For this review, use the dimensioned drawing (mm, ordinates from the lowest corner) and the shaded views. Give positions to 0.01 mm unless a question says otherwise; leave off trailing zeros. Loops run counter-clockwise (first coordinate to the right, second up) from the corner with the lowest first, then second, coordinate; pieces in that order, holes last. Notation, with made-up numbers: M -31.75,69.5 L -7.75,69.5 A29 cw -7.75,92.5 Z; hole C -13,9.5 d8. An arc over 180 degrees is marked long. Use CSV: the item, a comma, the result in double quotes.
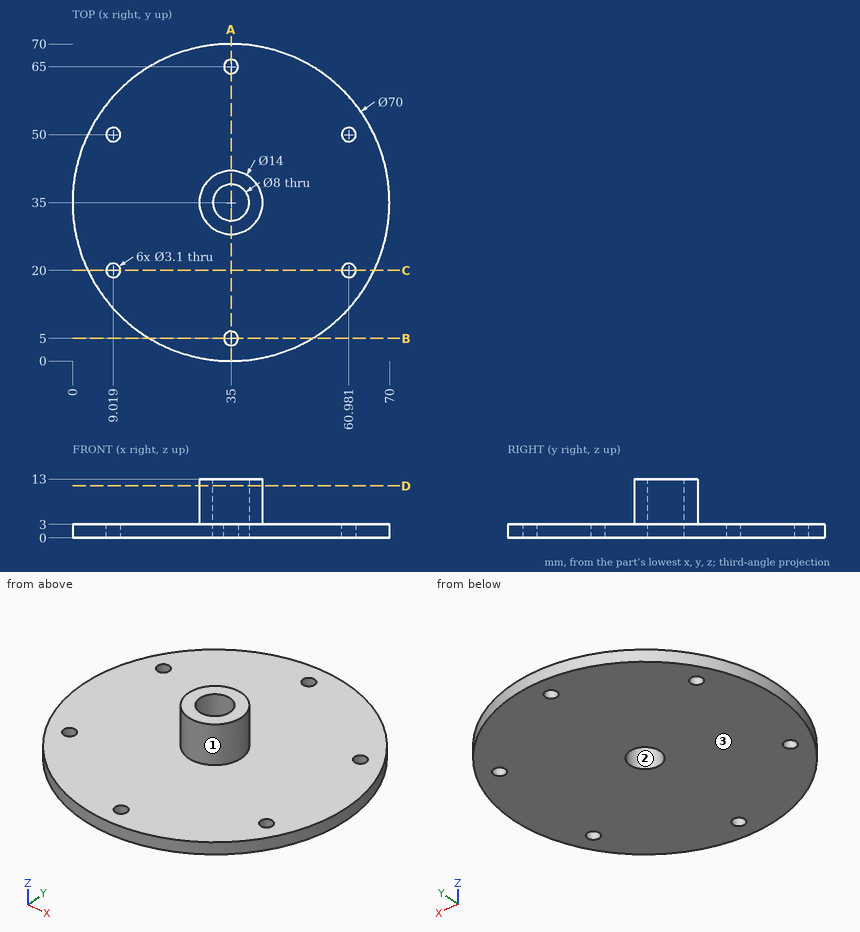
(1) We need section D-D on z = 11.5. State the section outline as (x, y) points.
A:
outline,"C 35,35 d14; hole C 35,35 d8"
(2) We need section C-C on y = 20. State the section outline as (x, z) points, then the cut area to 3 significant figures.
A:
outline,"M 3.38,0 L 7.47,0 L 7.47,3 L 3.38,3 Z; M 10.57,0 L 59.43,0 L 59.43,3 L 10.57,3 Z; M 62.53,0 L 66.62,0 L 66.62,3 L 62.53,3 Z"
area,"171 mm²"
(3) Clearance check with flat-ended pins moving along their axes: P1, Ø3, axis at x = 13, y = 37.5, coming from the -Z side; P2, Ø6, axis at x = 44.5, y = 55, coming from the +Z side; P3, Ø1.9, axis at x = 60.98, y = 20, coming from the -Z side; P4, Ø2, axis at x = 42, z = 2, coming from the +Y side. State where each tip first meets the part, or that it passes through.
A:
P1,"z = 0"
P2,"z = 3"
P3,"through"
P4,"y = 69.48"
(4) The part is to be moulded in two halves that separate along X. For the marked faces 1, 2 and 3, say which applies: released by +X, released by -X, zero draft, split by the parting line, or undercut.
A:
face 1,"split by the parting line"
face 2,"undercut"
face 3,"zero draft"
(5) Wall thickness on line 1 along Y through (x, z) = (35, 1.45); line 2 along Z through (x, y) = (38, 5.5); line 3 along X through (y, z) = (65, 1.9): over which ranges is each line inside the solid? List them lowest first. Write a range as [from, to].
A:
line 1,"[0, 3.45], [6.55, 31], [39, 63.45], [66.55, 70]"
line 2,"[0, 3]"
line 3,"[16.97, 33.45], [36.55, 53.03]"
(6) We need section A-A on x = 35. State the section outline as (y, z) points, then the cut area to 3 significant figures.
A:
outline,"M 0,0 L 3.45,0 L 3.45,3 L 0,3 Z; M 6.55,0 L 31,0 L 31,13 L 28,13 L 28,3 L 6.55,3 Z; M 39,0 L 63.45,0 L 63.45,3 L 42,3 L 42,13 L 39,13 Z; M 66.55,0 L 70,0 L 70,3 L 66.55,3 Z"
area,"227 mm²"
(7) We need section B-B on y = 5. State the section outline as (x, z) points.
A:
outline,"M 16.97,0 L 33.45,0 L 33.45,3 L 16.97,3 Z; M 36.55,0 L 53.03,0 L 53.03,3 L 36.55,3 Z"
